Source: CAD feature listing. Evaluate the final solid. Frame: model axes, mm. Give positions to 0.01 mm unless a question says otherwise; leave off trailing zeros. Order: outer loops, then holes, each group sorted by start corner. A loop starts at its lowest first (then second) coordinate and runs counter-clockwise, first axis right, second up. Notation, with made-up numbers: M 12,70.25 L 22,70.25 A28 cw 22,105.25 Z; hole C 83,83.5 d10. An arc over 180 degrees is marked long. Use CSV: the item, a comma, the result in double quotes. Start each with the question number.
Item 1: Section query A-A on y = -17. Return loops of the section in (x, z).
Item 2: Section query C-C on z = 9.5. Count the separate pieces of the cut face and the enclosed holes in it, and give its area (3 significant figures).
Item 3: Section query B-B on x = -36. Return loops of the section in (y, z), and give its area (3 significant figures).
Item 4: Ray query, probe 1 along X at (y, z) = (-57, 11.25); probe 2 along Y at (x, z) = (-3.5, 3.75). Return the intervals inside material, ascending. Write a range as from..to.
Item 5: First-contact query: pin 1 (4.5 mm diameter, centred on x = -114.3, y = 127, fed in from -Z) (3 decimals); pin 2 (6.5 mm diameter, centred on x = -114.3, y = -127, fed in from +Z); pin 3 (1.8 mm diameter, centred on x = 114.3, y = -127, fed in from +Z). Flat tips, straight axial feed; report the tip coordinate or a pass-through.
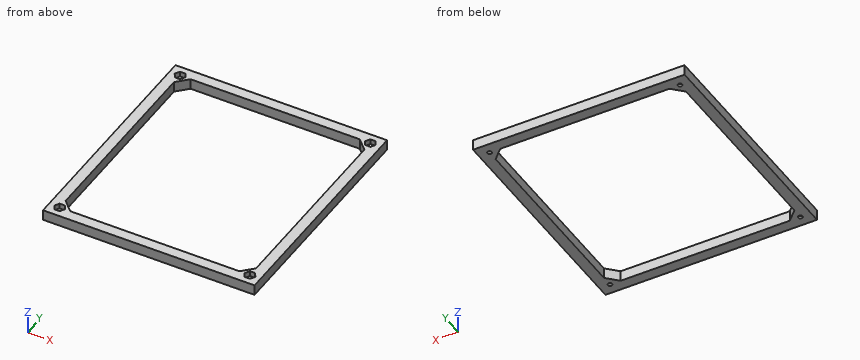
from build123d import *

# Parameters (mm, degrees)
F1_DEPTH = 12.7
F3_DEPTH = 6.35
F4_R     = 1.524
F5_DEPTH = 6.351
F6_R     = 2.54
F7_DEPTH = 3.175


with BuildPart() as f1:
    # F0 (on Top) → F1 (new body)
    with BuildSketch(Plane.XY):
        Polygon((127, 114.3), (127, 139.7), (101.6, 139.7), (-101.6, 139.7), (-127, 139.7), (-127, 114.3), (-127, -114.3), (-127, -139.7), (-101.6, -139.7), (101.6, -139.7), (127, -139.7), (127, -114.3), align=None)
        Polygon((-101.6, 127), (101.6, 127), (114.3, 114.3), (114.3, -114.3), (101.6, -127), (-101.6, -127), (-114.3, -114.3), (-114.3, 114.3), align=None, mode=Mode.SUBTRACT)
    extrude(amount=F1_DEPTH)

    # F2 (on face) → F3 (cut)
    with BuildSketch(Plane.XY.offset(12.7)):
        Polygon((111.125, -121.500739), (107.95, -127), (111.125, -132.499261), (117.475, -132.499261), (120.65, -127), (117.475, -121.500739), align=None)
        Polygon((-117.475, -132.499261), (-111.125, -132.499261), (-107.95, -127), (-111.125, -121.500739), (-117.475, -121.500739), (-120.65, -127), align=None)
        Polygon((-107.95, 127), (-111.125, 132.499261), (-117.475, 132.499261), (-120.65, 127), (-117.475, 121.500739), (-111.125, 121.500739), align=None)
        Polygon((120.65, 127), (117.475, 132.499261), (111.125, 132.499261), (107.95, 127), (111.125, 121.500739), (117.475, 121.500739), align=None)
    extrude(amount=-F3_DEPTH, mode=Mode.SUBTRACT)

    # F4 (on face) → F5 (cut, through all)
    with BuildSketch(Plane.XY.offset(6.35)):
        with Locations((-114.3, 127)):
            Circle(F4_R)
        with Locations((114.3, 127)):
            Circle(F4_R)
        with Locations((114.3, -127)):
            Circle(F4_R)
        with Locations((-114.3, -127)):
            Circle(F4_R)
    extrude(amount=-F5_DEPTH, mode=Mode.SUBTRACT)

    # F6 (on face) → F7 (cut)
    with BuildSketch(Plane(origin=(0, 0, 0), x_dir=(1, 0, 0), z_dir=(0, 0, -1))):
        with Locations((-114.3, 127)):
            Circle(F6_R)
        with Locations((114.3, 127)):
            Circle(F6_R)
        with Locations((-114.3, -127)):
            Circle(F6_R)
        with Locations((114.3, -127)):
            Circle(F6_R)
    extrude(amount=-F7_DEPTH, mode=Mode.SUBTRACT)


solid = f1.part
Verdict:
1,outline,"M -127,0 L -114.3,0 L -114.3,12.7 L -127,12.7 Z; M 114.3,0 L 127,0 L 127,12.7 L 114.3,12.7 Z"
2,separate pieces,"1"
2,enclosed holes,"5"
2,area,"12,800 mm2"
3,outline,"M -139.7,0 L -127,0 L -127,12.7 L -139.7,12.7 Z; M 127,0 L 139.7,0 L 139.7,12.7 L 127,12.7 Z"
3,area,"323 mm2"
4,probe 1,"-127..-114.3, 114.3..127"
4,probe 2,"-139.7..-127, 127..139.7"
5,pin 1,"z = 3.175"
5,pin 2,"z = 6.35"
5,pin 3,"through"
